Could you check a few things on this model? Use its own coordinates, in mm. A direction names the side the tool comes from. Round coordinates to 2 decimals unless told otherwise and drop trailing zeros. Write each loop counter-clockwise with the first axis right and the second up, starting at its lowest first coordinate (ties: lowest second). Pieces come first, ordered by that corner, then holes. Notation, with made-up numbers: (-36.5, 17) -> (20.5, 17) arc R27 ccw to (20.5, 51) -> close; hole circle Ø8 at (62.5, 62.5). An arc over 180 degrees is marked (long way). Answer in a Markdown table with one row per item.
from build123d import *

# Parameters (mm, degrees)
CROQUIS2_R              = 45
SALIENTE_EXTRUIR1_DEPTH = 2
CROQUIS3_R              = 43.25
CROQUIS3_R_2            = 41.75
SALIENTE_EXTRUIR2_DEPTH = 10
CROQUIS4_R              = 45
CROQUIS4_R_2            = 43.25
SALIENTE_EXTRUIR3_DEPTH = 5
CROQUIS6_R              = 12.56
CROQUIS6_R_2            = 10.56
SALIENTE_EXTRUIR4_DEPTH = 2.5
CROQUIS7_R              = 0.8
CORTAR_EXTRUIR1_DEPTH   = 65.420493634
SALIENTE_EXTRUIR5_DEPTH = 6
CROQUIS10_R             = 1.45
SALIENTE_EXTRUIR6_DEPTH = 4
CROQUIS11_W             = 19.7
CROQUIS11_H             = 18.7
SALIENTE_EXTRUIR7_DEPTH = 2
CROQUIS12_R             = 3.151866764
SALIENTE_EXTRUIR8_DEPTH = 2.5
REDONDEO1_R             = 9.25
REDONDEO2_R             = 0.7
REDONDEO4_R             = 5


# Some blends are built 0.0001 mm under size
with BuildPart() as part:
    # Croquis2 → Saliente-Extruir1 (new body)
    with BuildSketch(Plane(origin=(0, 0, 0), x_dir=(1, 0, 0), z_dir=(0, 1, 0))):
        with Locations(Location((0, 0, 0), (0, 0, 270))):
            Circle(CROQUIS2_R)
    extrude(amount=SALIENTE_EXTRUIR1_DEPTH)

    # Croquis3 → Saliente-Extruir2 (add)
    with BuildSketch(Plane(origin=(0, 2, 0), x_dir=(1, 0, 0), z_dir=(0, 1, 0))):
        with Locations(Location((0, 0, 0), (0, 0, 270))):
            Circle(CROQUIS3_R)
        with Locations(Location((0, 0, 0), (0, 0, 270))):
            Circle(CROQUIS3_R_2, mode=Mode.SUBTRACT)
    extrude(amount=SALIENTE_EXTRUIR2_DEPTH)

    # Croquis4 → Saliente-Extruir3 (add)
    with BuildSketch(Plane(origin=(0, 2, 0), x_dir=(1, 0, 0), z_dir=(0, 1, 0))):
        with Locations(Location((0, 0, 0), (0, 0, 270))):
            Circle(CROQUIS4_R)
        with Locations(Location((0, 0, 0), (0, 0, 270))):
            Circle(CROQUIS4_R_2, mode=Mode.SUBTRACT)
    extrude(amount=SALIENTE_EXTRUIR3_DEPTH)

    # Croquis6 → Saliente-Extruir4 (add)
    with BuildSketch(Plane(origin=(0, 2, 0), x_dir=(1, 0, 0), z_dir=(0, 1, 0))):
        with Locations(Location((0, 0, 0), (0, 0, 270))):
            Circle(CROQUIS6_R)
        with Locations(Location((0, 0, 0), (0, 0, 270))):
            Circle(CROQUIS6_R_2, mode=Mode.SUBTRACT)
    extrude(amount=SALIENTE_EXTRUIR4_DEPTH)

    # Croquis7 → Cortar-Extruir1 (cut, through all)
    with BuildSketch(Plane(origin=(0, 2, 0), x_dir=(1, 0, 0), z_dir=(0, 1, 0))):
        with Locations(Location((0, 7.075, 0), (0, 0, 270))):
            Circle(CROQUIS7_R)
        with Locations(Location((3.4, 7.075, 0), (0, 0, 270))):
            Circle(CROQUIS7_R)
        with Locations(Location((-3.4, 7.075, 0), (0, 0, 90))):
            Circle(CROQUIS7_R)
        with Locations(Location((7.075, 3.4, 0), (0, 0, 90))):
            Circle(CROQUIS7_R)
        with Locations(Location((7.075, 0, 0), (0, 0, 270))):
            Circle(CROQUIS7_R)
        with Locations(Location((7.075, -3.4, 0), (0, 0, 270))):
            Circle(CROQUIS7_R)
        with Locations(Location((3.4, -7.075, 0), (0, 0, 90))):
            Circle(CROQUIS7_R)
        with Locations(Location((0, -7.075, 0), (0, 0, 270))):
            Circle(CROQUIS7_R)
        with Locations(Location((-3.4, -7.075, 0), (0, 0, 270))):
            Circle(CROQUIS7_R)
        with Locations(Location((-7.075, -3.4, 0), (0, 0, 90))):
            Circle(CROQUIS7_R)
        with Locations(Location((-7.075, 0, 0), (0, 0, 270))):
            Circle(CROQUIS7_R)
        with Locations(Location((-7.075, 3.4, 0), (0, 0, 270))):
            Circle(CROQUIS7_R)
    extrude(amount=-CORTAR_EXTRUIR1_DEPTH, mode=Mode.SUBTRACT)

    # Croquis8 → Saliente-Extruir5 (add)
    with BuildSketch(Plane.XZ):
        Polygon((-7.25, 9.05), (14.75, 9.05), (14.75, -30.45), (-7.25, -30.45), (-7.25, -39.45), (23.75, -39.45), (23.75, 18.05), (-7.25, 18.05), align=None)
    extrude(amount=SALIENTE_EXTRUIR5_DEPTH)

    # Croquis10 → Saliente-Extruir6 (add)
    # profile 1 of 2: a face of its own
    with BuildSketch(Plane.ZY.offset(7.25)):
        with BuildLine():
            Line((9.75, -24.7), (9.75, -6))
            Line((9.75, -6), (17.25, -6))
            Line((17.25, -6), (17.25, -21.25))
            ThreePointArc((17.25, -21.25), (16.239518395, -23.689518395), (13.8, -24.7))
            Line((13.8, -24.7), (9.75, -24.7))
        make_face()
        with Locations((13.8, -11.25)):
            Circle(CROQUIS10_R, mode=Mode.SUBTRACT)
        with Locations(Location((13.8, -21.25, 0), (0, 0, 180))):
            Circle(CROQUIS10_R, mode=Mode.SUBTRACT)
    # profile 2 of 2: a face of its own
    with BuildSketch(Plane.ZY.offset(7.25)):
        with BuildLine():
            Line((-31.15, -24.7), (-31.15, -6))
            Line((-31.15, -6), (-38.65, -6))
            Line((-38.65, -6), (-38.65, -21.25))
            ThreePointArc((-38.65, -21.25), (-37.639518395, -23.689518395), (-35.2, -24.7))
            Line((-35.2, -24.7), (-31.15, -24.7))
        make_face()
        with Locations((-35.2, -21.25)):
            Circle(CROQUIS10_R, mode=Mode.SUBTRACT)
        with Locations(Location((-35.2, -11.25, 0), (0, 0, 180))):
            Circle(CROQUIS10_R, mode=Mode.SUBTRACT)
    extrude(amount=-SALIENTE_EXTRUIR6_DEPTH)

    # Croquis11 → Saliente-Extruir7 (add)
    with BuildSketch(Plane(origin=(23.75, 0, 0), x_dir=(0, 0, -1), z_dir=(1, 0, 0))):
        with Locations((21.3, -15.35)):
            Rectangle(CROQUIS11_W, CROQUIS11_H)
    extrude(amount=-SALIENTE_EXTRUIR7_DEPTH)

    # Croquis12 → Saliente-Extruir8 (add)
    with BuildSketch(Plane(origin=(23.75, 0, 0), x_dir=(0, 0, -1), z_dir=(1, 0, 0))):
        with Locations(Location((20.77, -16.25, 0), (0, 0, 180))):
            Circle(CROQUIS12_R)
    extrude(amount=SALIENTE_EXTRUIR8_DEPTH)

    # Redondeo1
    # the kernel refuses this fillet: 9.25 mm, written as the material it adds along each edge
    with BuildSketch(Plane(origin=(23.75, -6, -31.15), x_dir=(0, 0, -1), z_dir=(-1, 0, 0))) as redondeo1_piece_1:
        with BuildLine():
            CenterArc((9.25, 9.201086892), REDONDEO1_R, 180, 84.1051745)
            Line((0, 9.201086892), (0, 0))
            Line((0, 0), (8.3, 0))
        make_face()
    extrude(amount=2)
    with BuildSketch(Plane(origin=(23.75, -6, -11.45), x_dir=(0, 0, 1), z_dir=(-1, 0, 0))) as redondeo1_piece_2:
        with BuildLine():
            CenterArc((REDONDEO1_R, -REDONDEO1_R), REDONDEO1_R, 90, 90)
            Line((0, -REDONDEO1_R), (0, 0))
            Line((0, 0), (REDONDEO1_R, 0))
        make_face()
    extrude(amount=2)
    # the kernel refuses this fillet: 9.25 mm, written as the material it takes off along each edge
    with BuildSketch(Plane(origin=(46.875, -24.7, -31.15), x_dir=(0, 0, 1), z_dir=(-1, 0, 0)), Plane(origin=(46.875, -24.7, -11.45), x_dir=(0, 1, 0), z_dir=(-1, 0, 0))) as redondeo1_2_piece_1:
        with BuildLine():
            CenterArc((REDONDEO1_R, REDONDEO1_R), REDONDEO1_R, 180, 90)
            Line((0, REDONDEO1_R), (0, 0))
            Line((0, 0), (REDONDEO1_R, 0))
        make_face()
    extrude(amount=48.25, mode=Mode.SUBTRACT)

    # Redondeo2
    redondeo2_edges = [part.edges().sort_by_distance(p)[0] for p in [
        (-3.25, -6, -34.9),
        (-5.25, -6, -38.65),
        (-5.25, -6, -31.15),
        (-3.25, -6, 13.5),
        (-5.25, -6, 9.75),
        (-5.25, -6, 17.25),
    ]]
    fillet(redondeo2_edges, radius=REDONDEO2_R - 0.0001)  # a hair under: the kernel refuses the full size

    # Redondeo4
    # the kernel refuses this fillet: 5 mm, written as the material it takes off along each edge
    with BuildSketch(Plane(origin=(23.75, 0, -39.45), x_dir=(0, 0, 1), z_dir=(0, -1, 0))) as redondeo4_piece_1:
        with BuildLine():
            CenterArc((REDONDEO4_R, REDONDEO4_R), REDONDEO4_R, 180, 90)
            Line((0, REDONDEO4_R), (0, 0))
            Line((0, 0), (REDONDEO4_R, 0))
        make_face()
    extrude(amount=18.5, mode=Mode.SUBTRACT)


solid = part.part
1) Imagine slicing it at B-B, the plane z = -16. Please give me the cut outline in (x, y).
Findings:
| item | result |
|---|---|
| outline | (-42.06, 0) -> (14.75, 0) -> (14.75, -6) -> (21.75, -6) -> (21.75, -23.42) -> (23.75, -23.42) -> (23.75, 0) -> (42.06, 0) -> (42.06, 7) -> (40.18, 7) -> (40.18, 12) -> (38.56, 12) -> (38.56, 2) -> (-38.56, 2) -> (-38.56, 12) -> (-40.18, 12) -> (-40.18, 7) -> (-42.06, 7) -> close |
2) Imagine slicing it at A-A, the plane y = -11.25. Please give me the cut outline in (x, z), plus the area to 3 significant figures.
Findings:
| item | result |
|---|---|
| outline | (-7.25, -38.65) -> (-3.25, -38.65) -> (-3.25, -36.65) -> (-7.25, -36.65) -> close; (-7.25, -33.75) -> (-3.25, -33.75) -> (-3.25, -31.15) -> (-7.25, -31.15) -> close; (-7.25, 9.75) -> (-3.25, 9.75) -> (-3.25, 12.35) -> (-7.25, 12.35) -> close; (-7.25, 15.25) -> (-3.25, 15.25) -> (-3.25, 17.25) -> (-7.25, 17.25) -> close; (21.75, -32.04) -> (23.75, -32.04) -> (23.75, -10.54) -> (21.75, -10.54) -> close |
| area | 79.8 mm^2 |
3) Imagine slicing it at C-C, the plane x = -23. Please give me the cut outline in (y, z).
Findings:
| item | result |
|---|---|
| outline | (0, -38.68) -> (7, -38.68) -> (7, -36.63) -> (12, -36.63) -> (12, -34.84) -> (2, -34.84) -> (2, 34.84) -> (12, 34.84) -> (12, 36.63) -> (7, 36.63) -> (7, 38.68) -> (0, 38.68) -> close |
4) For faces 1 (the face through (-10.31, 3.23, -2.29)), 2 (the face through (-5, -16, -31.15)), 3 (the face through (-7.25, -9, 14)), 4 (the face through (-5, -16, 9.75)), 5 (the face through (-5, -14, 17.25)), which set-ups out of +Z, -Z, +X, -X, +Y, -Y let a thin tool reach every point of the face, with its end or its side?
Findings:
| item | result |
|---|---|
| face 1 | +Y |
| face 2 | -X, -Y |
| face 3 | +Z, -Z, -X, -Y |
| face 4 | +X, -X, -Y |
| face 5 | +Z, +X, -X, -Y |
5) Imagine slicing it at D-D, the plane x = -35. Please give me the cut outline in (y, z), plus the area to 3 significant figures.
Findings:
| item | result |
|---|---|
| outline | (0, -28.28) -> (7, -28.28) -> (7, -25.41) -> (12, -25.41) -> (12, -22.76) -> (2, -22.76) -> (2, 22.76) -> (12, 22.76) -> (12, 25.41) -> (7, 25.41) -> (7, 28.28) -> (0, 28.28) -> close |
| area | 195 mm^2 |
6) For pin 1 (6 mm diameter, centred on y = 6.5, z = -5.5, fed in from +X); pin 2 (8 mm diameter, centred on x = -25, z = 15.5, fed in from +Y); pin 3 (2.5 mm diameter, centred on y = -8, z = 15.5, fed in from -X); pin 4 (1.3 mm diameter, centred on x = 7.075, z = 0, fed in from -Y), each with a flat end and sliding along its axis, tell me the tip position at first contact or that it passes through.
Findings:
| item | result |
|---|---|
| pin 1 | stops at x = 44.93 |
| pin 2 | stops at y = 2 |
| pin 3 | stops at x = -7.25 |
| pin 4 | passes through |
7) Thinking about a two-plate mould opening in X: for faces 6 (the face through (-7.25, -12.2, -33.9)), 7 (the face through (8, -3, 18.05)), 8 (the face through (15, -6, -10)), 9 (the face through (3.77, 3.23, 11.98)), which applies, +X half, -X half, draft (parallel to the pull), parting line (faces both ways), or undercut?
Findings:
| item | result |
|---|---|
| face 6 | -X half |
| face 7 | draft |
| face 8 | undercut |
| face 9 | undercut |
8) Please list where these lines run through material, in increasing order: line 1 (X direction, y = 1.55, z = 0) (3 decimals); line 2 (Y direction, x = -6.35, z = 13.8); line 3 (X direction, y = 1.2, z = -3.4) (3 decimals).
Findings:
| item | result |
|---|---|
| line 1 | x = -45 to -7.875, -6.275 to 6.275, 7.875 to 45 |
| line 2 | y = -24.7 to -22.7, -19.8 to -12.7, -9.8 to 2 |
| line 3 | x = -44.871 to -7.875, -6.275 to 6.275, 7.875 to 44.871 |
